Build history of the part. All positions in model axes, mm. Face numbers are marked on the shaded views. Round coordinates to 2 decimals unless told otherwise and drop trailing zeros. Write each loop counter-clockwise with the first axis right and the second up, starting at its lowest first coordinate (ties: lowest second). Pieces come first, ordered by that corner, then holes.
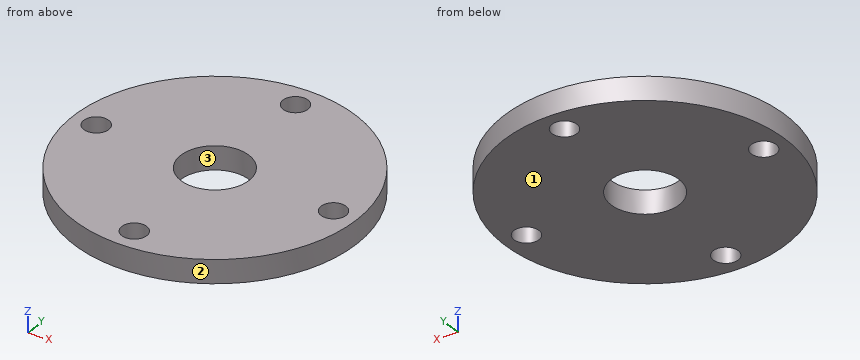
from build123d import *

# Parameters (mm, degrees)
SKETCH1_R           = 38.1
BOSS_EXTRUDE1_DEPTH = 6.35
SKETCH2_R           = 3.3782
CUT_EXTRUDE1_DEPTH  = 6.35
SKETCH3_R           = 9.2075
CUT_EXTRUDE2_DEPTH  = 6.35


with BuildPart() as part:
    # Sketch1 → Boss-Extrude1 (new body)
    with BuildSketch(Plane.XY):
        Circle(SKETCH1_R)
    extrude(amount=BOSS_EXTRUDE1_DEPTH)

    # Sketch2 → Cut-Extrude1 (cut)
    with BuildSketch(Plane.XY.offset(6.35)):
        with Locations((0, 31.75)):
            Circle(SKETCH2_R)
        with Locations((31.75, 0)):
            Circle(SKETCH2_R)
        with Locations((0, -31.75)):
            Circle(SKETCH2_R)
        with Locations((-31.75, 0)):
            Circle(SKETCH2_R)
    extrude(amount=-CUT_EXTRUDE1_DEPTH, mode=Mode.SUBTRACT)

    # Sketch3 → Cut-Extrude2 (cut)
    with BuildSketch(Plane.XY.offset(6.35)):
        Circle(SKETCH3_R)
    extrude(amount=-CUT_EXTRUDE2_DEPTH, mode=Mode.SUBTRACT)


solid = part.part
1) Pin check, flat tips, straight feed: pin 1 Ø3 at (x, z) = (-25.5, 2) entering from -Y; pin 2 Ø1 at (y, z) = (17.5, 2.5) entering from +X; pin 3 Ø1 at (y, z) = (-16, 5) entering from +X. Stop position of each tip, or through.
Results:
pin 1: stops at y = -29.59
pin 2: stops at x = 34.1
pin 3: stops at x = 34.8
2) Slice it at C-C (y = -31.75). Write the cut outline in (x, z).
Results:
outline: (-21.06, 0) - (-3.38, 0) - (-3.38, 6.35) - (-21.06, 6.35) - close; (3.38, 0) - (21.06, 0) - (21.06, 6.35) - (3.38, 6.35) - close
3) Wall check: L1, parallel to Y at x = 0, z = 2; L2, parallel to Y at x = 2.5, z = 1.75; L3, parallel to X at y = 2, z = 2.5. Give the ranges that are in metal, low to high.
Results:
L1: y = -38.1 to -35.13, -28.37 to -9.21, 9.21 to 28.37, 35.13 to 38.1
L2: y = -38.02 to -34.02, -29.48 to -8.86, 8.86 to 29.48, 34.02 to 38.02
L3: x = -38.05 to -34.47, -29.03 to -8.99, 8.99 to 29.03, 34.47 to 38.05
4) Slice it at D-D (z = 5.25). Count the separate pieces of the cut face and the enclosed holes in it, plus the area to 3 significant figures.
Results:
separate pieces: 1
enclosed holes: 5
area: 4,150 mm2
5) Mould opens along Y. For the marked faces 1, 2 and 3 say: released by +Y, released by -Y, zero draft, split by the parting line, or undercut.
Results:
face 1: zero draft
face 2: split by the parting line
face 3: undercut
6) Slice it at A-A (y = 0). Write the cut outline in (x, z).
Results:
outline: (-38.1, 0) - (-35.13, 0) - (-35.13, 6.35) - (-38.1, 6.35) - close; (-28.37, 0) - (-9.21, 0) - (-9.21, 6.35) - (-28.37, 6.35) - close; (9.21, 0) - (28.37, 0) - (28.37, 6.35) - (9.21, 6.35) - close; (35.13, 0) - (38.1, 0) - (38.1, 6.35) - (35.13, 6.35) - close
